```python
from build123d import *

# Parameters (mm, degrees)
SKETCH1_W           = 110
SKETCH1_H           = 100
BOSS_EXTRUDE1_DEPTH = 10
SKETCH2_R           = 2
CUT_EXTRUDE1_DEPTH  = 115.564392374
SKETCH3_R           = 2.5
CUT_EXTRUDE2_DEPTH  = 10


with BuildPart() as part:
    # Sketch1 → Boss-Extrude1 (new body)
    with BuildSketch(Plane(origin=(0, 0, 0), x_dir=(1, 0, 0), z_dir=(0, 1, 0))):
        Rectangle(SKETCH1_W, SKETCH1_H)
    extrude(amount=BOSS_EXTRUDE1_DEPTH)

    # Sketch2 → Cut-Extrude1 (cut, through all)
    with BuildSketch(Plane.XY.offset(50)):
        with Locations((-50, 5)):
            Circle(SKETCH2_R)
        with Locations(Location((50, 5, 0), (0, 0, 180))):
            Circle(SKETCH2_R)
    extrude(amount=-CUT_EXTRUDE1_DEPTH, mode=Mode.SUBTRACT)

    # Sketch3 → Cut-Extrude2 (cut)
    with BuildSketch(Plane(origin=(0, 10, 0), x_dir=(1, 0, 0), z_dir=(0, 1, 0))):
        with Locations(Location((-45, -37, 0), (0, 0, 270))):
            Circle(SKETCH3_R)
        with Locations(Location((45, -37, 0), (0, 0, 90))):
            Circle(SKETCH3_R)
        with Locations(Location((45, 37, 0), (0, 0, 270))):
            Circle(SKETCH3_R)
        with Locations(Location((-45, 37, 0), (0, 0, 90))):
            Circle(SKETCH3_R)
    extrude(amount=-CUT_EXTRUDE2_DEPTH, mode=Mode.SUBTRACT)


solid = part.part
```
Model file for the job. Use its own axes, mm. Give positions to 0.01 mm unless a question says otherwise; leave off trailing zeros. Write each loop counter-clockwise with the first axis right and the second up, starting at its lowest first coordinate (ties: lowest second). Pieces come first, ordered by that corner, then holes. Notation, with made-up numbers: M 72,80 L 90,80 A34 cw 90,113 Z; hole C 64,87 d7. An arc over 180 degrees is marked long. Use a Markdown table: item, result.
1) Pull direction X, two halves, no side cores. Call faces 1 (the flat face through (55, 5, 1)), 2 (the cylindrical face through (-45.96, 5.07, 39.31)), 3 (the flat face through (-1, 0, -1)), 4 (the flat face through (-55, 5, 1)): +X half, -X half, draft (parallel to the pull), parting line (faces both ways), or undercut.
Responses:
| item | result |
|---|---|
| face 1 | +X half |
| face 2 | undercut |
| face 3 | draft |
| face 4 | -X half |
2) Pin check, flat tip, straight feed: pin 1 (4.5 mm diameter, centred on x = 45, z = 37, fed in from +Y). Stop position of the tip, or through.
Responses:
| item | result |
|---|---|
| pin 1 | passes through |
3) Cut at A-A (z = -37). List the corners of the cut face in (x, y), and give its area (3 significant figures).
Responses:
| item | result |
|---|---|
| outline | M -55,0 L -47.5,0 L -47.5,10 L -55,10 Z; M -42.5,0 L 42.5,0 L 42.5,10 L -42.5,10 Z; M 47.5,0 L 55,0 L 55,10 L 47.5,10 Z; hole C -50,5 d4; hole C 50,5 d4 |
| area | 975 mm2 |
4) Drill centre lines: line 1 (X direction, y = 4.5, z = 3.5); line 2 (Y direction, x = -50, z = 27); line 3 (X direction, y = 0.5, z = 35). Where is each one in solid material? Low to high. Write a range as from..to.
Responses:
| item | result |
|---|---|
| line 1 | x = -55..-51.94, -48.06..48.06, 51.94..55 |
| line 2 | y = 0..3, 7..10 |
| line 3 | x = -55..-46.5, -43.5..43.5, 46.5..55 |
5) Cut at D-D (z = 44). List the corners of the cut face in (x, y).
Responses:
| item | result |
|---|---|
| outline | M -55,0 L 55,0 L 55,10 L -55,10 Z; hole C -50,5 d4; hole C 50,5 d4 |
6) Cut at C-C (x = 50). List the corners of the cut face in (y, z).
Responses:
| item | result |
|---|---|
| outline | M 0,-50 L 3,-50 L 3,50 L 0,50 Z; M 7,-50 L 10,-50 L 10,50 L 7,50 Z |
7) Cut at B-B (y = 5). List the corners of the cut face in (x, z).
Responses:
| item | result |
|---|---|
| outline | M -55,-50 L -52,-50 L -52,50 L -55,50 Z; M -48,-50 L 48,-50 L 48,50 L -48,50 Z; M 52,-50 L 55,-50 L 55,50 L 52,50 Z; hole C -45,-37 d5; hole C -45,37 d5; hole C 45,-37 d5; hole C 45,37 d5 |
